```python
from build123d import *

# Parameters (mm, degrees)
SKETCH1_W           = 60
SKETCH1_H           = 50
BOSS_EXTRUDE1_DEPTH = 10
SKETCH2_W           = 15
SKETCH2_H           = 30
REVOLVE1_ANGLE      = 120


with BuildPart() as part:
    # Sketch1 → Boss-Extrude1 (new, symmetric)
    with BuildSketch(Plane.XY):
        with Locations((0, 15)):
            Rectangle(SKETCH1_W, SKETCH1_H)
    extrude(amount=BOSS_EXTRUDE1_DEPTH, both=True)

    # Sketch2 → Revolve1 (revolve)
    with BuildSketch(Plane.XY):
        with Locations((12.5, 15)):
            Rectangle(SKETCH2_W, SKETCH2_H)
    revolve(axis=Axis((0, 0, 0), (0, -1, 0)), revolution_arc=REVOLVE1_ANGLE)


solid = part.part
```
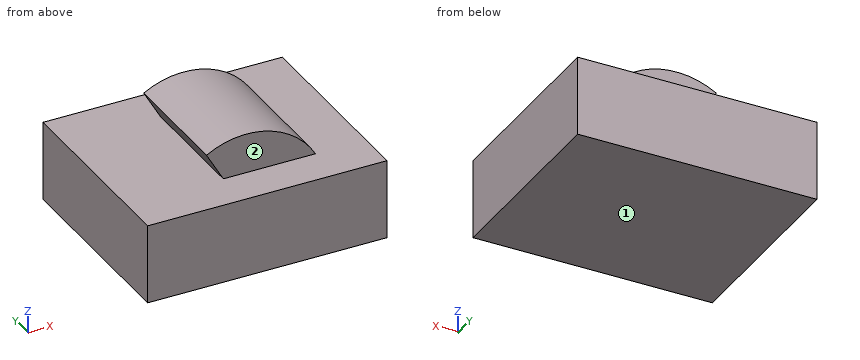
Could you check a few things on this model? Use its own coordinates, in mm. Face numbers are marked on the shaded views. A direction names the side the tool comes from. Coordinates: 2 decimals unless noted, no trailing zeros. Write each loop counter-clockwise with the first axis right and the second up, starting at its lowest first coordinate (ties: lowest second). Pieces come first, ordered by that corner, then holes. Notation, with made-up numbers: (39.25, 89.25) -> (93.25, 89.25) arc R7 cw to (93.25, 102.25) -> close; hole circle Ø8 at (-2, -6.75). An arc over 180 degrees is marked (long way). Write item = value, one per line. Start each with the question number.
(1) I want a section at D-D (x = -16.5). Please give me the cut outline in (y, z).
(2) Will these pins go through, and if not, where does the flat tip stop? pin 1 (10 mm diameter, centred on x = -1, z = 12.5, fed in from +Y); pin 2 (8 mm diameter, centred on x = 10, y = 7.5, fed in from +Z); pin 3 (8 mm diameter, centred on x = 9, z = 16, fed in from +Y).
(3) I want a section at B-B (y = 24). Please give me the cut outline in (x, z).
(4) I want a section at C-C (z = 14.5). Please give me the cut outline in (x, y).
(5) I want a section at A-A (x = 12). Please give me the cut outline in (y, z), plus the area to 3 significant figures.
(6) Which directions (+Z, -Z, +X, -X, +Y, -Y) give clear straight access to the entire face, cutting with the end or side of a thin tool? Please do the marked faces 1 and 2.
(7) I need wall thicknesses on line 1 (Z direction, x = 20.5, y = 17); line 2 (Y direction, x = -7.5, z = 17.5); line 3 (Z direction, x = 13, y = 20). Which ranges of each line are inside material? Lowest first, please. Write a range as [from, to].
Result set:
q1.outline = (-10, -10) -> (40, -10) -> (40, 10) -> (-10, 10) -> close
q2.pin_1 = 40
q2.pin_2 = 19.08
q2.pin_3 = 30
q3.outline = (-30, -10) -> (30, -10) -> (30, 10) -> (17.32, 10) arc R20 ccw to (-10, 17.32) -> (-5.77, 10) -> (-30, 10) -> close
q4.outline = (-8.37, 0) -> (13.77, 0) -> (13.77, 30) -> (-8.37, 30) -> close
q5.outline = (-10, -10) -> (40, -10) -> (40, 10) -> (30, 10) -> (30, 16) -> (0, 16) -> (0, 10) -> (-10, 10) -> close
q5.area = 1,180 mm2
q6.face_1 = -Z, +X, -X, +Y, -Y
q6.face_2 = +Z, +X, -X, -Y
q7.line_1 = [-10, 10]
q7.line_2 = [0, 30]
q7.line_3 = [-10, 15.2]
